Autodesk Inventor part; units mm, degrees
ref_plane "Start Plane" through (0, 0, 0) normal (0, 0, 1) x (1, 0, 0)
ref_plane "End Plane" through (0, 0, 210) normal (0, 0, 1) x (1, 0, 0)
ref_plane "Work Plane4" through (12.7, 0, 0) normal (0, 0.018, -0.9998) x (1, 0, 0)
ref_plane "Start Plane" through (0, 0, 0) normal (0, 0, 1) x (1, 0, 0)
ref_plane "End Plane" through (0, 0, 210) normal (0, 0, 1) x (1, 0, 0)
sketch "Sketch" plane through (0, 0, 0) normal (0, 0, 1) x (1, 0, 0)
  line L0 (25.4, 0) -> (0, 0)
  line L1 (0, 0) -> (0, 25.4)
  line L2 (0, 25.4) -> (1.651, 25.4)
  line L3 (3.175, 23.876) -> (3.175, 6.477)
  line L4 (6.477, 3.175) -> (23.876, 3.175)
  line L5 (25.4, 1.651) -> (25.4, 0)
  line L6 (0, -11.0414) -> (0, 31.5385) construction
  line L7 (-11.0414, 0) -> (31.5385, 0) construction
  arc A0 (3.175, 6.477) -> (6.477, 3.175) centre (6.477, 6.477) ccw
  arc A1 (3.175, 23.876) -> (1.651, 25.4) centre (1.651, 23.876) ccw
  arc A2 (25.4, 1.651) -> (23.876, 3.175) centre (23.876, 1.651) ccw
  line L8 (0, 40.0545) -> (0, -19.5574) construction
  line L9 (-19.5574, 0) -> (40.0545, 0) construction
  point P0 (3.175, 25.4)
  point P1 (3.175, 3.175)
  point P2 (25.4, 3.175)
  dimension "d0" = 25.4
  dimension "d1" = 25.4
  dimension "d2" = 3.175
  dimension "d3" = 3.175
  dimension "d10" = 0
  dimension "d11" = 0
  dimension "d14" = 3.302
  dimension "d15" = 1.524
extrude "Body" add sketch "Sketch" along normal up to surface (210 mm away) from surface at 0
sketch "Sketch3" plane through (0, 0, 0) normal (0, 0, 1) x (1, 0, 0)
  line L0 (0, 0) -> (10, 0)
ref_plane "Work Plane3" through (0, 0, 0) normal (0, -1, 0) x (1, 0, 0)
ref_plane "Work Plane4" through (12.7, 0, 0) normal (0, 0.018, -0.9998) x (1, 0, 0)
split "Split1" plane through (12.7, 0, 0) removes the side toward (0, 0.018, -0.9998)
ref_plane "Work Plane8" through (0, 12.7, 210) normal (0.7071, 0, 0.7071) x (0.7071, 0, -0.7071)
split "Split2" plane through (0, 12.7, 210) removes the side toward (0.7071, 0, 0.7071)
sketch "Sketch4" plane through (0, 0, 0) normal (0, -1, 0) x (1, 0, 0)
  line L0 (-2, 0) -> (12, 0)
  line L1 (-2, 210) -> (12, 210)
  dimension "d17" = 210
equation "\"d0\" = G_H"
equation "\"d1\" = G_H"
equation "\"d2\" = G_T"
equation "\"d3\" = G_T"
equation "\"d14\" = G_IR"
equation "\"d15\" = G_ER"
equation "\"d4\" = G_L"
equation "\"G_H\" = 25.4"
equation "\"G_T\" = 3.175"
equation "\"G_ER\" = 1.524"
equation "\"G_IR\" = 3.302"
equation "\"G_L\" = d17"
equation "\"ex\" = 0"
equation "\"G_OFFSET_START\" = 0"
equation "\"G_OFFSET_END\" = 0"
equation "\"d13\" = G_OFFSET_END + B_L"
equation "\"B_L\" = 210"
properties part number "AISC - L 1 x 1 x 1/8 - 8.268" material "Steel, Mild"
Can you work these out from the model? Positions are in its coordinate system, mm. A direction names the side the tool comes from. Round coordinates to 2 decimals unless told otherwise and drop trailing zeros. Loops run counter-clockwise (first coordinate to the right, second up) from the corner with the lowest first, then second, coordinate; pieces in that order, holes last. Notation, with made-up numbers: (74.5, 62) - (121.5, 62) arc R10 cw to (121.5, 69) - close; hole circle Ø9 at (85, 53.25). An arc over 180 degrees is marked (long way). Use CSV: the item, a comma, the result in double quotes. Start each with the question number.
1) If we section it at A-A on z = 145: Write out the boundary of the cut face in (x, y) (3 decimals), plus the area to 3 significant figures.
2) If we section it at B-B on y = 12.75: Write out the boundary of the cut face in (x, z) (3 decimals), plus the area to 3 significant figures.
3) If we section it at C-C on x = 10.5: Write out the boundary of the cut face in (y, z) (3 decimals), plus the area to 3 significant figures.
4) Please list where these lines run through material, in increasing order: probe 1 along X at (y, z) = (12, 51) (3 decimals); probe 2 along Y at (x, z) = (4.75, 148). Write a range as [from, to].
5) For pin 1 Ø1.5 at (y, z) = (10, 188.5) entering from +X (3 decimals); pin 2 Ø10 at (x, z) = (19.5, 53.5) entering from +Y (3 decimals), each with a flat end and sliding along its axis, tell me the tip position at first contact or that it passes through.
6) For faces 1 (the flat face through (13, 0, 104)), 2 (the flat face through (15, 3.175, 100)), which set-ups out of +Z, -Z, +X, -X, +Y, -Y let a thin tool reach every point of the face, with its end or its side?
Geometry results:
1,outline,"(0, 0) - (25.4, 0) - (25.4, 1.651) arc R1.524 ccw to (23.876, 3.175) - (6.477, 3.175) arc R3.302 cw to (3.175, 6.477) - (3.175, 23.876) arc R1.524 ccw to (1.651, 25.4) - (0, 25.4) - close"
1,area,"153 mm2"
2,outline,"(0, 0.23) - (3.175, 0.23) - (3.175, 206.825) - (0, 210) - close"
2,area,"661 mm2"
3,outline,"(0, 0) - (3.175, 0.057) - (3.175, 199.5) - (0, 199.5) - close"
3,area,"633 mm2"
4,probe 1,"x = [0, 3.175]"
4,probe 2,"y = [0, 3.66]"
5,pin 1,"stops at x = 3.175"
5,pin 2,"stops at y = 3.175"
6,face 1,"+Z, -Z, +X, -X, -Y"
6,face 2,"+Z, -Z, +X, +Y"
